from build123d import *

# Parameters (mm, degrees)
PAD_DEPTH = 5


with BuildPart() as part:
    # Sketch → Pad (new body)
    with BuildSketch(Plane.XY):
        Polygon((0, 40), (13, 40), (13, 14), (30, 30), (40, 30), (40, 20), (18.75, 0), (0, 0), align=None)
    extrude(amount=PAD_DEPTH)


with BuildPart() as part_1:
    # Body placement: moved
    add(part.part.moved(Location((-16, 0, 0))))


solid = part_1.part
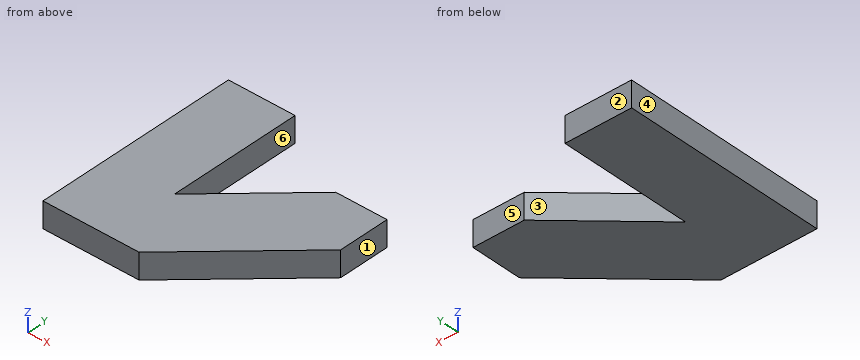
Geometry: final body of the model. Coordinates: model frame, mm. Face numbers are marked on the shaded views. A direction names the side the tool comes from. Give positions to 0.01 mm unless a question says otherwise; leave off trailing zeros. Write each loop counter-clockwise with the first axis right and the second up, starting at its lowest first coordinate (ties: lowest second). Pieces come first, ordered by that corner, then holes. Notation, with made-up numbers: M 46.25,35 L 66.25,35 A27 cw 66.25,70 Z; hole C 49,63 d5. An arc over 180 degrees is marked long. Answer in a Markdown table with one row per item. Add a question column.
(1) First-contact query: pin 1 (12 mm diameter, centred on x = -2, y = 9, fed in from -Z); pin 2 (2.5 mm diameter, centred on x = 21, z = 3.5, fed in from +Y). Flat tips, straight axial feed; report the tip coordinate or a pass-through.
(2) Section D-D on y = 20.5. Return loops of the section in (x, z).
(3) Section B-B on z = 0.6. Return loops of the section in (x, y).
(4) Ray query, line 1 (X direction, y = 33, z = 0.45); line 2 (X direction, y = 17.5, z = 4.5); line 3 (X direction, y = 21, z = 4.05). Return the intervals inside material, ascending.
(5) Mould query, pull axis X, two halves, no side actions, for the marked faces 1, 2 and 3. Classes: +X half, -X half, draft (parallel to the pull), parting line (faces both ways), or undercut.
(6) Section A-A on y = 26. Return loops of the section in (x, z), and give its area (3 significant figures).
(7) Reachability of the marked faces 4, 5 and 6 from +Z, -Z, +X, -X, +Y, -Y: full face, straight path, thin tool, end or side. Return the list, or none.
(8) Section C-C on x = 11. Return loops of the section in (y, z).
Result set:
| question | item | result |
|---|---|---|
| 1 | pin 1 | stops at z = 0 |
| 1 | pin 2 | stops at y = 30 |
| 2 | outline | M -16,0 L -3,0 L -3,5 L -16,5 Z; M 3.91,0 L 24,0 L 24,5 L 3.91,5 Z |
| 3 | outline | M -16,0 L 2.75,0 L 24,20 L 24,30 L 14,30 L -3,14 L -3,40 L -16,40 Z |
| 4 | line 1 | x = -16 to -3 |
| 4 | line 2 | x = -16 to -3, 0.72 to 21.34 |
| 4 | line 3 | x = -16 to -3, 4.44 to 24 |
| 5 | face 1 | +X half |
| 5 | face 2 | draft |
| 5 | face 3 | undercut |
| 6 | outline | M -16,0 L -3,0 L -3,5 L -16,5 Z; M 9.75,0 L 24,0 L 24,5 L 9.75,5 Z |
| 6 | area | 136 mm^2 |
| 7 | face 4 | +Z, -Z, -X, +Y, -Y |
| 7 | face 5 | +Z, -Z, +X, +Y |
| 7 | face 6 | +Z, -Z, +Y |
| 8 | outline | M 7.76,0 L 27.18,0 L 27.18,5 L 7.76,5 Z |
